Autodesk Inventor part; units mm, degrees
ref_plane "Work Plane1" through (0, 0, 10) normal (0, 0, 1) x (1, 0, 0)
ref_plane "YZ Plane" through (0, 0, 0) normal (1, 0, 0) x (0, 1, 0)
ref_plane "XZ Plane" through (0, 0, 0) normal (0, 1, 0) x (-1, 0, 0)
ref_plane "Work Plane1" through (0, 0, 10) normal (0, 0, 1) x (1, 0, 0)
sketch "Sketch1" plane through (0, 0, 10) normal (0, 0, 1) x (1, 0, 0)
  line L0 (-4.0299, -0.3538) -> (-2.2322, 1.4439) construction
  arc A0 (-1.4439, 2.2322) -> (-2.2322, 1.4439) centre (-0.9299, 0.9299) ccw construction
  line L1 (-1.4439, 2.2322) -> (0.3538, 4.0299) construction
  line L2 (-37.8299, 42.8299) -> (-37.8299, 37.8299) construction
  line L3 (-37.8299, 37.8299) -> (-42.9208, 37.8299) construction
  line L4 (-37.8299, 42.2137) -> (-37.8299, 45.8299) construction
  line L5 (-37.8299, 45.8299) -> (-4.0299, 45.8299) construction
  line L6 (-4.0299, 45.8299) -> (-4.0299, 42.2137) construction
  line L7 (-4.0299, 4.0299) -> (0.3538, 4.0299)
  circle A1 centre (-20.9299, 20.9299) radius 17.5
  line L8 (-20.9299, 58.9723) -> (17.1124, 20.9299) construction
  line L9 (17.1124, 20.9299) -> (-20.9299, -17.1124) construction
  line L10 (-20.9299, -17.1124) -> (-58.9723, 20.9299) construction
  line L11 (-58.9723, 20.9299) -> (-20.9299, 58.9723) construction
  line L12 (-20.9299, 58.9723) -> (-20.9299, -17.1124) construction
  line L13 (17.1124, 20.9299) -> (-58.9723, 20.9299) construction
  line L14 (-20.9299, 58.9723) -> (32.8701, 58.9723) construction
  line L15 (-43.4299, 43.4299) -> (1.5701, 43.4299) construction
  line L16 (1.5701, 43.4299) -> (1.5701, -1.5701) construction
  line L17 (1.5701, -1.5701) -> (-43.4299, -1.5701) construction
  line L18 (-43.4299, -1.5701) -> (-43.4299, 43.4299) construction
  line L19 (-43.4299, 43.4299) -> (1.5701, -1.5701) construction
  line L20 (1.5701, 43.4299) -> (-43.4299, -1.5701) construction
  line L21 (-43.4299, 5.3876) -> (-43.4299, 36.4723)
  line L22 (-43.4299, 36.4723) -> (-36.4723, 43.4299)
  line L23 (-36.4723, 43.4299) -> (-5.3876, 43.4299)
  line L24 (-5.3876, 43.4299) -> (1.5701, 36.4723)
  line L25 (1.5701, 36.4723) -> (1.5701, 5.3876)
  line L26 (1.5701, 5.3876) -> (-5.3876, -1.5701)
  line L27 (-5.3876, -1.5701) -> (-36.4723, -1.5701)
  line L28 (-36.4723, -1.5701) -> (-43.4299, 5.3876)
  line L29 (-4.0299, 42.2137) -> (-37.8299, 42.2137)
  line L30 (-4.0299, -0.3538) -> (-4.0299, 4.0299)
  circle A2 centre (-20.9299, 20.9299) radius 1.5
  line L31 (-10.9299, 10.9299) -> (-30.9299, 10.9299) construction
  line L32 (-30.9299, 10.9299) -> (-30.9299, 30.9299) construction
  line L33 (-30.9299, 30.9299) -> (-10.9299, 30.9299) construction
  line L34 (-10.9299, 30.9299) -> (-10.9299, 10.9299) construction
  line L35 (-10.9299, 10.9299) -> (-30.9299, 30.9299) construction
  line L36 (-30.9299, 10.9299) -> (-10.9299, 30.9299) construction
  circle A3 centre (-30.9299, 30.9299) radius 1.4
  circle A4 centre (-30.9299, 10.9299) radius 1.4
  circle A5 centre (-10.9299, 10.9299) radius 1.4
  line L37 (-45.8299, 37.8299) -> (-42.0723, 37.8299) construction
  line L38 (-42.1723, 37.7299) -> (-45.8299, 37.7299)
  line L39 (-45.8299, 37.7299) -> (-45.8299, 4.1299)
  line L40 (-45.8299, 4.1299) -> (-42.1723, 4.1299)
  line L41 (-42.1723, 4.1299) -> (-42.1723, 37.7299)
  line L42 (-45.8299, 4.0299) -> (-42.0723, 4.0299) construction
  line L43 (-45.8299, 37.8299) -> (-42.0723, 37.8299)
  line L44 (-37.7299, 45.8299) -> (-4.1299, 45.8299)
  line L45 (-4.1299, 45.8299) -> (-4.1299, 42.1723)
  line L46 (-4.1299, 42.1723) -> (-37.7299, 42.1723)
  line L47 (-37.7299, 42.1723) -> (-37.7299, 45.8299)
  line L48 (0.4701, 37.8299) -> (0.4701, 4.0299) construction
  line L49 (0.4701, 4.0299) -> (3.9701, 4.0299) construction
  line L50 (3.9701, 37.8299) -> (3.9701, 4.0299) construction
  line L51 (0.4701, 37.8299) -> (3.9701, 37.8299) construction
  line L52 (-45.8299, -3.9701) -> (-4.0299, -3.9701) construction
  line L53 (0.3124, 37.7299) -> (3.9701, 37.7299)
  line L54 (3.9701, 37.7299) -> (3.9701, 4.1299)
  line L55 (3.9701, 4.1299) -> (0.3124, 4.1299)
  line L56 (0.3124, 4.1299) -> (0.3124, 37.7299)
  line L57 (-4.1713, -0.3538) -> (-37.7299, -0.3538)
  line L58 (-37.7299, -0.3538) -> (-37.7299, -3.9701)
  line L59 (-37.7299, -3.9701) -> (-4.1713, -3.9701)
  line L60 (-4.1713, -3.9701) -> (-4.1713, -0.3538)
  point P0 (-37.8299, 4.0299)
  dimension "d18" = 53.8
  dimension "d19" = 45
  dimension "d20" = 53.8
  dimension "d21" = 45
  dimension "d22" = 45
  dimension "d30" = 20
  dimension "d31" = 20
  dimension "d32" = 2.8
  dimension "d33" = 2.8
  dimension "d34" = 2.8
  dimension "d35" = 3
  dimension "d36" = 0.1
  dimension "d37" = 0.1
  dimension "d38" = 0.1
  dimension "d39" = 0.1
extrude "Extrusion1" add sketch "Sketch1" along normal blind 3 contours L30 L26 L57 L28 L41 L22 L46 L24 L56 L7 | L7 L26 L30 | L56 L24 L25 L26 | L26 L25 L24 L53 L54 L55 | L60 L59 L58 L57 L28 L27 L26 | L26 L27 L28 L57 | L46 L22 L29 L24 | L24 L29 L45 | L40 L39 L38 L22 L21 L28 | L28 L21 L22 L41 | L29 L22 L23 L24 | L24 L23 L22 L29 L47 L44 L45 | L47 L29 L22 | A1 | A2 | A3 | A4 | A5
sketch "Skizze4" plane through (0, 0, 13) normal (0, 0, 1) x (1, 0, 0)
  line L0 (-37.7299, 42.1723) -> (-42.1723, 37.7299)
  line L1 (-42.1723, 37.7299) -> (-45.8299, 37.7299)
  line L2 (-45.8299, 37.7299) -> (-45.8299, 4.1299) construction
  line L3 (-45.8299, 4.1299) -> (-42.1723, 4.1299)
  line L4 (-42.1723, 4.1299) -> (-37.6885, -0.3538)
  line L5 (-37.6885, -0.3538) -> (-37.7299, -0.3538)
  line L6 (-37.7299, -0.3538) -> (-37.7299, -3.9701)
  line L7 (-37.7299, -3.9701) -> (-4.1713, -3.9701) construction
  line L8 (-4.1713, -3.9701) -> (-4.1713, -0.3538)
  line L9 (-4.1713, -0.3538) -> (0.3124, 4.1299)
  line L10 (0.3124, 4.1299) -> (3.9701, 4.1299)
  line L11 (3.9701, 4.1299) -> (3.9701, 37.7299) construction
  line L12 (3.9701, 37.7299) -> (0.3124, 37.7299)
  line L13 (0.3124, 37.7299) -> (-4.1299, 42.1723)
  line L14 (-4.1299, 42.1723) -> (-4.1299, 45.8299)
  line L15 (-4.1299, 45.8299) -> (-37.7299, 45.8299) construction
  line L16 (-37.7299, 45.8299) -> (-37.7299, 42.1723)
  line L17 (-37.9299, 46.0299) -> (-3.9299, 46.0299) construction
  line L18 (-3.9299, 46.0299) -> (-3.9299, 42.2551)
  line L19 (-3.9299, 42.2551) -> (0.3953, 37.9299)
  line L20 (0.3953, 37.9299) -> (4.1701, 37.9299)
  line L21 (4.1701, 37.9299) -> (4.1701, 3.9299) construction
  line L22 (4.1701, 3.9299) -> (0.3953, 3.9299)
  line L23 (0.3953, 3.9299) -> (-3.9713, -0.4367)
  line L24 (-3.9713, -0.4367) -> (-3.9713, -4.1701)
  line L25 (-3.9713, -4.1701) -> (-37.9299, -4.1701) construction
  line L26 (-37.9299, -4.1701) -> (-37.9299, -0.3953)
  line L27 (-37.9299, -0.3953) -> (-42.2551, 3.9299)
  line L28 (-42.2551, 3.9299) -> (-46.0299, 3.9299)
  line L29 (-46.0299, 3.9299) -> (-46.0299, 37.9299) construction
  line L30 (-46.0299, 37.9299) -> (-42.2551, 37.9299)
  line L31 (-42.2551, 37.9299) -> (-37.9299, 42.2551)
  line L32 (-37.9299, 42.2551) -> (-37.9299, 46.0299)
  line L33 (-45.8299, 37.7299) -> (-45.8299, 37.9299)
  line L34 (-4.1299, 45.8299) -> (-37.7299, 45.8299)
  line L35 (-37.7299, 45.8299) -> (-37.9299, 45.8299)
  line L36 (-4.1299, 45.8299) -> (-3.9299, 45.8299)
  line L37 (3.9701, 37.7299) -> (3.9701, 37.9299)
  line L38 (3.9701, 4.1299) -> (3.9701, 37.7299)
  line L39 (3.9701, 4.1299) -> (3.9701, 3.9299)
  line L40 (-4.1713, -3.9701) -> (-3.9713, -3.9701)
  line L41 (-37.7299, -3.9701) -> (-37.9299, -3.9701)
  line L42 (-45.8299, 4.1299) -> (-45.8299, 3.9299)
  point P0 (0, 0)
  dimension "d40" = 0.2
extrude "IM_offset" add sketch "Skizze4" against normal up to surface (3 mm away)
ref_plane "Arbeitsebene5" through (-20.9299, 3.9299, 10) normal (1, 0, 0) x (0, 0, -1)
ref_plane "Arbeitsebene6" through (-37.9299, 20.9299, 10) normal (0, 1, 0) x (1, 0, 0)
sketch "Skizze36" plane through (0, 0, 10) normal (0, 0, -1) x (-1, 0, 0)
  line L0 (-13.9301, 20.9299) -> (55.7899, 20.9299)
  line L1 (20.9299, -13.9301) -> (20.9299, 55.7899)
  line L2 (19.9299, 21.9299) -> (39.9299, 21.9299)
  line L3 (39.9299, 21.9299) -> (39.9299, 1.9299)
  line L4 (39.9299, 1.9299) -> (19.9299, 1.9299)
  line L5 (19.9299, 1.9299) -> (19.9299, 21.9299)
  line L6 (39.9299, 1.9299) -> (27.9299, 1.9299)
  line L7 (27.9299, 1.9299) -> (27.9299, 13.9299)
  line L8 (27.9299, 13.9299) -> (39.9299, 13.9299)
  line L9 (39.9299, 13.9299) -> (39.9299, 1.9299)
  point P0 (0, 0)
  point P1 (39.9299, 13.9299)
  point P2 (39.9299, 20.9299)
  point P3 (20.9299, 20.9299)
  point P4 (20.9299, 1.9299)
  point P5 (27.9299, 1.9299)
  dimension "d197" = 20
  dimension "d198" = 20
  dimension "d199" = 1
  dimension "d200" = 1
  dimension "d201" = 12
  dimension "d202" = 12
extrude "Extrusion32" add sketch "Skizze36" along normal blind 20 contours L5 L2 L1 L0 | L0 L1 L4 L5 | L1 L2 L3 L0 | L0 L3 L8 L7 L4 L1
ref_plane "Arbeitsebene10" through (0, 0, -4) normal (0, 0, 1) x (1, 0, 0)
sketch "Skizze37" plane through (0, 0, -4) normal (0, 0, 1) x (1, 0, 0)
  line L0 (-19.9299, 1.3901) -> (-19.9299, 21.9308)
  line L1 (-19.9299, 21.9308) -> (-19.9299, 13.3467)
  line L2 (-19.9299, 13.3467) -> (-21.9299, 13.3467)
  line L3 (-21.9299, 13.3467) -> (-21.9299, 17.9308)
  line L4 (-21.9299, 21.9308) -> (-19.9299, 21.9308)
  line L5 (-40.9299, 1.3901) -> (-19.9299, 1.3901)
  line L6 (-22.807, 4.3901) -> (-22.807, 7.3107)
  line L7 (-23.807, 7.3107) -> (-23.807, 4.3901)
  line L8 (-22.807, 7.3107) -> (-22.807, 9.7285) construction
  line L9 (-22.807, 9.7285) -> (-20.1457, 10.6003) construction
  line L10 (-20.1457, 10.6003) -> (-19.9299, 13.3467) construction
  spline S0 degree 3 poles (-22.807, 7.3107) (-22.807, 9.7285) (-20.1457, 10.6003) (-19.9299, 13.3467) knots 1 1 1 1 2 2 2 2
  spline S1 degree 3 poles (-23.807, 7.3107) (-23.807, 11.2353) (-23.1457, 11.6741) (-21.9299, 13.3467) knots 1 1 1 1 2 2 2 2
  line L11 (-23.807, 7.3107) -> (-23.807, 11.2353) construction
  line L12 (-23.807, 11.2353) -> (-23.1457, 11.6741) construction
  line L13 (-23.1457, 11.6741) -> (-21.9299, 13.3467) construction
  line L14 (-21.9299, 21.9308) -> (-21.9299, 19.9308)
  line L15 (-23.9299, 19.9308) -> (-28.9019, 19.9308)
  line L16 (-28.9019, 19.9308) -> (-28.9019, 21.9308)
  line L17 (-28.9019, 21.9308) -> (-21.9299, 21.9308)
  line L18 (-19.9299, 21.9308) -> (-29.9299, 11.9308) construction
  line L19 (-28.9019, 21.9308) -> (-28.9019, 19.9308)
  line L20 (-31.2605, 21.715) -> (-28.9019, 21.9308) construction
  spline S2 degree 3 poles (-34.55, 19.0538) (-32.1323, 19.0538) (-31.2605, 21.715) (-28.9019, 21.9308) knots 1 1 1 1 2 2 2 2
  line L21 (-34.55, 19.0538) -> (-32.1323, 19.0538) construction
  line L22 (-32.1323, 19.0538) -> (-31.2605, 21.715) construction
  line L23 (-30.1867, 18.715) -> (-28.9019, 19.9308) construction
  spline S3 degree 3 poles (-34.55, 18.0538) (-30.6255, 18.0538) (-30.1867, 18.715) (-28.9019, 19.9308) knots 1 1 1 1 2 2 2 2
  line L24 (-34.55, 18.0538) -> (-30.6255, 18.0538) construction
  line L25 (-30.6255, 18.0538) -> (-30.1867, 18.715) construction
  line L26 (-37.4706, 19.0538) -> (-34.55, 19.0538)
  line L27 (-34.55, 18.0538) -> (-37.4706, 18.0538)
  line L28 (-40.4706, 18.0538) -> (-40.4706, 19.0538)
  line L29 (-22.807, 4.3901) -> (-23.807, 4.3901)
  line L30 (-37.4706, 18.0538) -> (-37.4706, 19.0538)
  arc A0 (-21.9299, 17.9308) -> (-23.9299, 19.9308) centre (-23.9299, 17.9308) ccw
  line L31 (-19.9299, 1.9299) -> (-19.9299, 21.9299)
  point P0 (0, 0)
  point P1 (-22.807, 1.3901)
  point P2 (-40.4706, 21.9308)
  point P3 (-19.9299, 13.3467)
  dimension "d206" = 2
  dimension "d207" = 2
  dimension "d208" = 1
  dimension "d209" = 3
  dimension "d210" = 3
  dimension "d211" = 2
  dimension "d214" = 0
extrude "Extrusion33" cut sketch "Skizze37" along normal mid plane 2
ref_plane "Arbeitsebene11" through (-19.9299, 21.9299, 10) normal (0.7071, -0.7071, 0) x (0, 0, -1)
sketch "Skizze38" plane through (-39.9299, 13.9299, 10) normal (-1, 0, 0) x (0, 0, 1)
  line L0 (-13, 8) -> (-15, 8)
  line L1 (-15, 4.1239) -> (-13, 4.1239)
  line L2 (-15, 5.1239) -> (-13, 5.1239)
  circle A0 centre (-13, 4.6008) radius 0.75
  point P0 (-10, -13.9299)
  dimension "d215" = 1.5
extrude "Extrusion34" cut sketch "Skizze38" against normal blind 5
mirror "Spiegeln3" about plane through (-19.9299, 21.9299, 10) normal (0.7071, -0.7071, 0) of "Extrusion34"
sketch "Skizze39" plane through (0, 0, -3) normal (0, 0, -1) x (-1, 0, 0)
  line L0 (39.9299, 13.9299) -> (39.9299, 21.9299)
  line L1 (39.9299, 21.9299) -> (19.9299, 21.9299)
  line L2 (19.9299, 21.9299) -> (19.9299, 1.9299)
  line L3 (19.9299, 1.9299) -> (27.9299, 1.9299)
  line L4 (27.9299, 1.9299) -> (27.9299, 13.9299)
  line L5 (27.9299, 13.9299) -> (39.9299, 13.9299)
  line L6 (19.9299, 21.9299) -> (20.4299, 21.9299)
  line L7 (20.4299, 21.9299) -> (20.4299, 21.4299)
  line L8 (20.4299, 21.4299) -> (19.9299, 21.4299)
  line L9 (19.9299, 21.4299) -> (19.9299, 21.9299)
  point P0 (0, 0)
  dimension "d218" = 0.5
  dimension "d219" = 0.5
extrude "Extrusion35" add sketch "Skizze39" along normal up to surface (2 mm away) contours L7 L8 L2 L1
properties part number "20_Cube_Insert_Lightsheet_Flowcube_rectangular_v3"
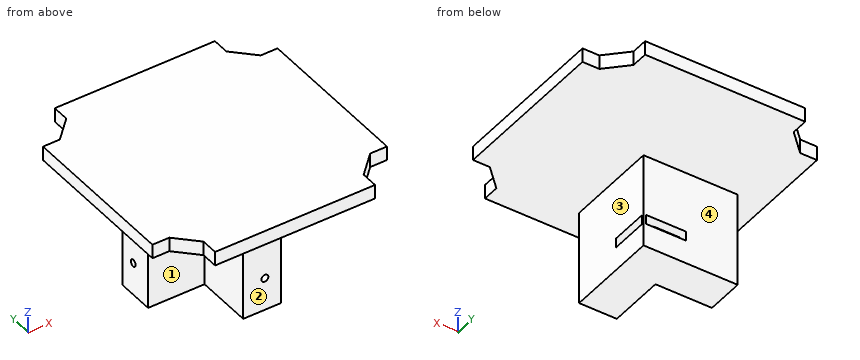
Geometry check sheet. Reference: the model listing, model coordinates, mm. Face numbers are marked on the shaded views. A direction names the side the tool comes from. Coordinates: 2 decimals unless noted, no trailing zeros. Write each loop counter-clockwise with the first axis right and the second up, starting at its lowest first coordinate (ties: lowest second). Pieces come first, ordered by that corner, then holes. Notation, with made-up numbers: M 41.5,26.25 L 81.5,26.25 A12 ccw 81.5,36.25 Z; hole C 77.5,23.5 d1. An arc over 180 degrees is marked long. One line per item, written item: value. Start each with the question number.
(1) Sectioned sample at A-A, the plane x = -16. Enter the section's corners in (y, z), and give its area (3 significant figures).
(2) Depth check by flat-ended pin: pin 1 (5 mm diameter, centred on x = -39, y = 2, fed in from -Z); pin 2 (0.6 mm diameter, centred on x = -27, z = -4, fed in from +Y); pin 3 (6 mm diameter, centred on y = 8.5, z = -4, fed in from +X). Enter the tip coordinate at first touch or a pass-through.
(3) Sectioned sample at B-B, the plane z = -8.5. Enter the section's corners in (x, y), and give its area (3 significant figures).
(4) Scan lines: line 1 along X through (y, z) = (5.6, -3); line 2 along Y through (x, z) = (-38.5, -3); line 3 along X through (y, z) = (21.5, 9). Record each from-to range of solid material in increasing order. Write a range as [from, to].
(5) Sectioned sample at C-C, the plane y = 32. Enter the section's corners in (x, z), and give its area (3 significant figures).
(6) Tool access check on the marked faces 1, 2, 3 and 4. Record the directions out of +Z, -Z, +X, -X, +Y, -Y that give a thin tool (end or side, any length) a straight path to the whole face; none if there is none.
Filled sheet:
1. outline: M -3.97,10 L 45.83,10 L 45.83,13 L -3.97,13 Z
1. area: 149 mm²
2. pin 1: z = 10
2. pin 2: y = 19.93
2. pin 3: x = -19.93
3. outline: M -39.93,13.93 L -27.93,13.93 L -27.93,1.93 L -19.93,1.93 L -19.93,21.93 L -39.93,21.93 Z
3. area: 256 mm²
4. line 1: [-27.93, -24.08], [-22.58, -19.93]
4. line 2: [13.93, 17.78], [19.28, 21.93]
4. line 3: [-39.93, -19.93]
5. outline: M -45.83,10 L 3.97,10 L 3.97,13 L -45.83,13 Z
5. area: 149 mm²
6. face 1: -Z, -X, -Y
6. face 2: -Z, +X, -X, -Y
6. face 3: -Z, +X, +Y, -Y
6. face 4: -Z, +X, -X, +Y
